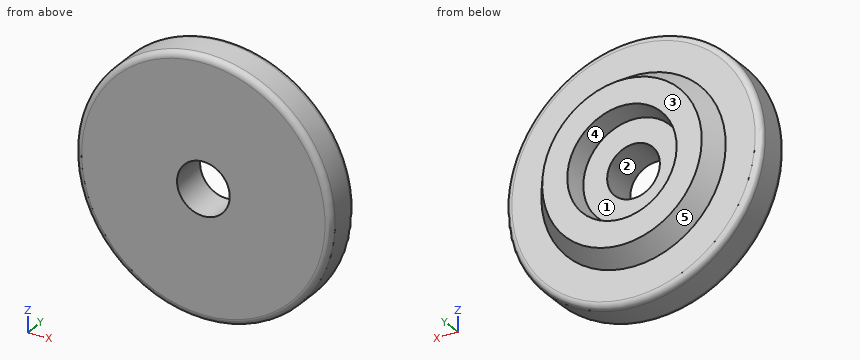
from build123d import *


with BuildPart() as part:
    # Sketch1 → Revolve1 (revolve)
    with BuildSketch(Plane.XY, mode=Mode.PRIVATE) as revolve1_sk:
        with BuildLine():
            Line((2.1, 0), (2.1, 3))
            Line((2.1, 3), (4, 3))
            Line((4, 3), (4.359369746, 4.5))
            Line((4.359369746, 4.5), (6.359369746, 4.5))
            Line((6.359369746, 4.5), (7.347987035, 3))
            Line((7.347987035, 3), (9.7, 3))
            ThreePointArc((9.7, 3), (10.053553391, 2.853553391), (10.2, 2.5))
            Line((10.2, 2.5), (10.2, 0.5))
            ThreePointArc((10.2, 0.5), (10.053553391, 0.146446609), (9.7, 0))
            Line((9.7, 0), (2.1, 0))
        make_face()
    revolve(revolve1_sk.sketch.rotate(Axis((0, 0, 0), (0, 1, 0)), 90), axis=Axis((0, 0, 0), (0, 1, 0)))


solid = part.part
CAD build for the part. Positions are in the model's coordinates, mm. Face numbers are marked on the shaded views. A direction names the side the tool comes from. Give positions to 0.01 mm unless a question says otherwise; leave off trailing zeros. Write each loop counter-clockwise with the first axis right and the second up, starting at its lowest first coordinate (ties: lowest second). Pieces come first, ordered by that corner, then holes. Notation, with made-up numbers: M 27.25,-10 L 86.25,-10 A26 ccw 86.25,8 Z; hole C 46,62.5 d11. An arc over 180 degrees is marked long. Put each result on its own line as item: value. Start each with the question number.
(1) Flat gauge pins, fed straight in: pin 1 Ø4 at (x, z) = (-1, -1.5) entering from +Y; pin 2 Ø10 at (x, z) = (-4.5, -6.5) entering from +Y; pin 3 Ø2 at (y, z) = (1, 2) entering from -X. Where does each tip first touch, or does it go through?
(2) Band-saw the part on B-B, the plane x = 0. Write the cut outline in (y, z), and give its area (3 significant figures).
(3) Band-saw the part on A-A, the plane z = 0. Write the cut outline in (x, y), and give its area (3 significant figures).
(4) Mould opens along Z. For the marked faces 3, 4 and 5 say: +Z half, -Z half, draft (parallel to the pull), parting line (faces both ways), or undercut.
(5) Probe L1, parallel to X at y = 0.8, z = 0; L2, parallel to Y at x = -6.5, z = 6.5; L3, parallel to X at y = 0.7, z = -1.5. List the from-to ranges inside material, lowest first.
(6) Band-saw the part on C-C, the plane y = 1.85. Write the cut outline in (x, z), and give its area (3 significant figures).
(7) Band-saw the part on D-D, the plane y = 3.4. Write the cut outline in (x, z).
(8) Which spindle directions (+Z, -Z, +X, -X, +Y, -Y) get a long thin tool onto all of the face, cutting with end or side? Do the marked faces 1 and 2. Say none if no direction does.
Response values:
1. pin 1: stops at y = 3
1. pin 2: stops at y = 4.5
1. pin 3: stops at x = -10.15
2. outline: M 0,-9.7 A0.5 ccw 0.5,-10.2 L 2.5,-10.2 A0.5 ccw 3,-9.7 L 3,-7.35 L 4.5,-6.36 L 4.5,-4.36 L 3,-4 L 3,-2.1 L 0,-2.1 Z; M 0,2.1 L 3,2.1 L 3,4 L 4.5,4.36 L 4.5,6.36 L 3,7.35 L 3,9.7 A0.5 ccw 2.5,10.2 L 0.5,10.2 A0.5 ccw 0,9.7 Z
2. area: 56.4 mm2
3. outline: M -10.2,0.5 A0.5 ccw -9.7,0 L -2.1,0 L -2.1,3 L -4,3 L -4.36,4.5 L -6.36,4.5 L -7.35,3 L -9.7,3 A0.5 ccw -10.2,2.5 Z; M 2.1,0 L 9.7,0 A0.5 ccw 10.2,0.5 L 10.2,2.5 A0.5 ccw 9.7,3 L 7.35,3 L 6.36,4.5 L 4.36,4.5 L 4,3 L 2.1,3 Z
3. area: 56.4 mm2
4. face 3: draft
4. face 4: undercut
4. face 5: parting line
5. L1: x = -10.2 to -2.1, 2.1 to 10.2
5. L2: y = 0 to 3
5. L3: x = -10.09 to -1.47, 1.47 to 10.09
6. outline: C 0,0 d20.4; hole C 0,0 d4.2
6. area: 313 mm2
7. outline: C 0,0 d14.17; hole C 0,0 d8.19
8. face 1: +Y
8. face 2: +Y, -Y
